Solid Edge part; units mm, degrees
sketch "Sketch1" plane through (0, 0, 0) normal (0, 0, 1) x (1, 0, 0)
  circle A0 centre (0, 0) radius 19
extrude "Protrusion1" add sketch "Sketch1" along normal blind 30
hole "Bohrung_1" at (0, 0, 30) direction (0, 0, -1) diameter 12 end through all
hole "Bohrung_2" at (0, 0, 30) direction (0, 0, -1) diameter 21 depth 24
chamfer "Fase_1" distance 1 angle 45 1 edges at (0, 10.5, 30)
chamfer "Fase_2" distance 5 angle 20 1 edges at (-19, 0, 30) measured on face at (10.5144, 15.8255, 24.7)
properties material "Aluminium, 1350"
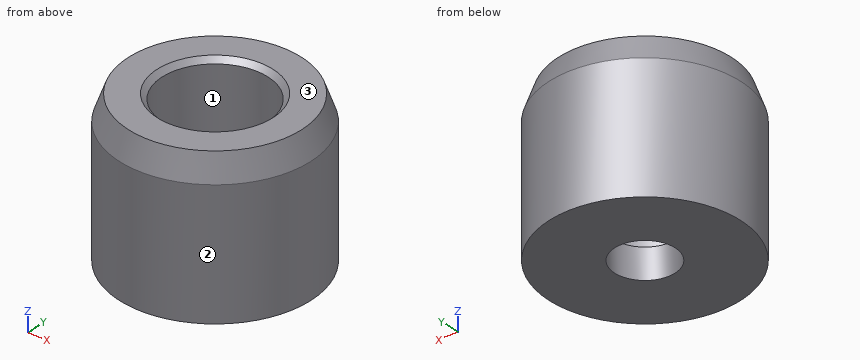
Input: part model. Units: mm. Frame: model coordinates. Face numbers are marked on the shaded views. Coordinates: 2 decimals unless noted, no trailing zeros. Write each loop counter-clockwise with the first axis right and the second up, starting at its lowest first coordinate (ties: lowest second). Pieces come first, ordered by that corner, then holes. Notation, with made-up numbers: M 60,22.5 L 64,22.5 A15 ccw 64,46.5 Z; hole C 46,41 d4. An arc over 180 degrees is marked long. Answer as a JSON object with one key per item and string values. Group by question number.
(1) Section D-D on z = 3.75. Output: boundary loops of the cut face in (x, y).
(2) Contact query for flat-ended pins moving along their axis: P1, Ø8, axis at x = 12.5, z = 7, coming from the +Y side; P2, Ø1, axis at y = 12.5, z = 5.5, coming from the +X side; P3, Ø3, axis at y = -8, z = 3, coming from the +X side. Output: stop coordinate, or through.
(3) Mould query, pull axis Y, two halves, no side actions, for the marked faces 1, 2 and 3. Classes: pulls with the +Y half, pulls with the -Y half, needs draft (parallel to the pull), parting line crosses it, or undercut.
(4) Section A-A on x = 0. Output: boundary loops of the cut face in (y, z).
(5) Ray query, line 1 along Y through (x, z) = (0, 23.5); line 2 along Y through (x, z) = (-5, 19.5); line 3 along Z through (x, y) = (-4, 9.5). Return the intervals inside material, ascending. Write a range as [from, to].
(6) Section C-C on z = 15.5. Output: boundary loops of the cut face in (x, y).
Result set:
{
 "1": {"outline": "C 0,0 d38; hole C 0,0 d12"},
 "2": {"P1": "stops at y = 16.99", "P2": "stops at x = 14.73", "P3": "stops at x = 17.85"},
 "3": {"face 1": "undercut", "face 2": "parting line crosses it", "face 3": "needs draft"},
 "4": {"outline": "M -19,0 L -6,0 L -6,6 L -10.5,6 L -10.5,29 L -11.5,30 L -17.18,30 L -19,25 Z; M 6,0 L 19,0 L 19,25 L 17.18,30 L 11.5,30 L 10.5,29 L 10.5,6 L 6,6 Z"},
 "5": {"line 1": "y = [-19, -10.5], [10.5, 19]", "line 2": "y = [-18.33, -9.23], [9.23, 18.33]", "line 3": "z = [0, 6]"},
 "6": {"outline": "C 0,0 d38; hole C 0,0 d21"}
}
